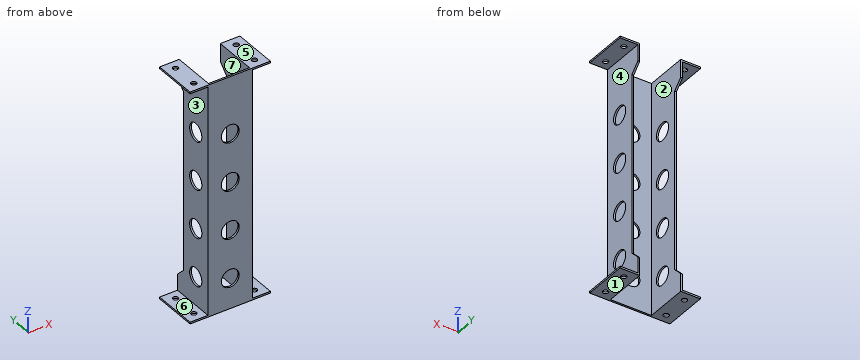
```python
from build123d import *

# Parameters (mm, degrees)
SKETCH1_W               = 25
SKETCH1_H               = 130
BOSS_EXTRUDE1_DEPTH     = 1
SKETCH2_W               = 1
SKETCH2_H               = 130
BOSS_EXTRUDE2_DEPTH     = 24
SKETCH3_W               = 1
SKETCH3_H               = 25
BOSS_EXTRUDE3_DEPTH     = 10
SKETCH4_W               = 1
SKETCH4_H               = 25
BOSS_EXTRUDE4_DEPTH     = 10
SKETCH5_R               = 5
CUT_EXTRUDE1_DEPTH      = 2
SKETCH10_R              = 1.5
CUT_EXTRUDE3_DEPTH      = 131
CUT_EXTRUDE4_DEPTH      = 11
CUT_EXTRUDE4_DEPTH_BACK = 36
SKETCH9_R               = 5
CUT_EXTRUDE2_DEPTH      = 36


with BuildPart() as part:
    # Sketch1 → Boss-Extrude1 (new body)
    with BuildSketch(Plane(origin=(0, 0, 0), x_dir=(1, 0, 0), z_dir=(0, 1, 0))):
        Rectangle(SKETCH1_W, SKETCH1_H)
    extrude(amount=BOSS_EXTRUDE1_DEPTH)

    # Sketch2 → Boss-Extrude2 (add)
    with BuildSketch(Plane(origin=(0, 1, 0), x_dir=(1, 0, 0), z_dir=(0, 1, 0))):
        with Locations((12, 0)):
            Rectangle(SKETCH2_W, SKETCH2_H)
        with Locations((-12, 0)):
            Rectangle(SKETCH2_W, SKETCH2_H)
    extrude(amount=BOSS_EXTRUDE2_DEPTH)

    # Sketch3 → Boss-Extrude3 (add)
    with BuildSketch(Plane(origin=(12.5, 0, 0), x_dir=(0, 0, -1), z_dir=(1, 0, 0))):
        with Locations((-64.5, 12.5)):
            Rectangle(SKETCH3_W, SKETCH3_H)
        with Locations((64.5, 12.5)):
            Rectangle(SKETCH3_W, SKETCH3_H)
    extrude(amount=BOSS_EXTRUDE3_DEPTH)

    # Sketch4 → Boss-Extrude4 (add)
    with BuildSketch(Plane.ZY.offset(12.5)):
        with Locations((-64.5, 12.5)):
            Rectangle(SKETCH4_W, SKETCH4_H)
        with Locations((64.5, 12.5)):
            Rectangle(SKETCH4_W, SKETCH4_H)
    extrude(amount=BOSS_EXTRUDE4_DEPTH)

    # Sketch5 → Cut-Extrude1 (cut, through all)
    with BuildSketch(Plane(origin=(0, 1, 0), x_dir=(1, 0, 0), z_dir=(0, 1, 0))):
        with Locations((0, -33)):
            Circle(SKETCH5_R)
        with Locations((0, -6)):
            Circle(SKETCH5_R)
        with Locations((0, 21)):
            Circle(SKETCH5_R)
        with Locations((0, 48)):
            Circle(SKETCH5_R)
    extrude(amount=-CUT_EXTRUDE1_DEPTH, mode=Mode.SUBTRACT)

    # Sketch10 → Cut-Extrude3 (cut, through all)
    with BuildSketch(Plane.XY.offset(65)):
        with Locations((17, 20)):
            Circle(SKETCH10_R)
        with Locations((17, 5)):
            Circle(SKETCH10_R)
        with Locations((-17, 20)):
            Circle(SKETCH10_R)
        with Locations((-17, 5)):
            Circle(SKETCH10_R)
    extrude(amount=-CUT_EXTRUDE3_DEPTH, mode=Mode.SUBTRACT)

    # Sketch11 → Cut-Extrude4 (cut, two sides)
    with BuildSketch(Plane(origin=(12.5, 0, 0), x_dir=(0, 0, -1), z_dir=(1, 0, 0))) as cut_extrude4_sk:
        Polygon((0, 25), (-55, 25), (-50, 20), (0, 20), align=None)
        Polygon((55, 25), (0, 25), (0, 20), (50, 20), align=None)
    extrude(amount=CUT_EXTRUDE4_DEPTH, mode=Mode.SUBTRACT)
    extrude(cut_extrude4_sk.sketch, amount=-CUT_EXTRUDE4_DEPTH_BACK, mode=Mode.SUBTRACT)

    # Sketch9 → Cut-Extrude2 (cut, through all)
    with BuildSketch(Plane(origin=(12.5, 0, 0), x_dir=(0, 0, -1), z_dir=(1, 0, 0))):
        with Locations((-33, 10)):
            Circle(SKETCH9_R)
        with Locations((-6, 10)):
            Circle(SKETCH9_R)
        with Locations((21, 10)):
            Circle(SKETCH9_R)
        with Locations((48, 10)):
            Circle(SKETCH9_R)
    extrude(amount=-CUT_EXTRUDE2_DEPTH, mode=Mode.SUBTRACT)


solid = part.part
```
Design review of the part built by this model. Coordinates are the model's own, in mm. Face numbers are marked on the shaded views. A direction names the side the tool comes from. Give positions to 0.01 mm unless a question says otherwise; leave off trailing zeros. Loops run counter-clockwise (first coordinate to the right, second up) from the corner with the lowest first, then second, coordinate; pieces in that order, holes last. Notation, with made-up numbers: M 69,32.25 L 126,32.25 A22 cw 126,54.25 Z; hole C 23,73.5 d1. An arc over 180 degrees is marked long. Return JSON: item names as keys, results as strings. Group by question number.
Item 1: Insertion check: pin 1 Ø0.5 at (x, z) = (-12, 3) entering from +Y; pin 2 Ø8 at (y, z) = (6, 10.5) entering from -X; pin 3 Ø8 at (y, z) = (6.5, -19) entering from +X; pin 4 Ø4 at (x, y) = (-17, 20) entering from +Z. Each pin has a flat end and moves straight along its axis. Give the tip position at first contact, or say it passes through.
Item 2: We need section C-C (z = -21). Give the boundary of the cut face in (x, y).
Item 3: Mouldability with a two-part tool opening along Z and no side actions: class the marked faces 1, 2 and 3 as released by +Z, released by -Z, zero draft, split by the parting line, or undercut.
Item 4: We need section A-A (y = 23.25). Give the boundary of the cut face in (x, z).
Item 5: For probe 1 along Y at (x, z) = (17, 64.3); probe 2 along Z at (x, y) = (0, 0.45); probe 3 along X at (y, z) = (21, 59.5), list the stretches that pass through material, from the lowest coordinate up.
Item 6: We need section B-B (x = 0). Give the boundary of the cut face in (y, z).
Item 7: We need section D-D (z = 44). Give the boundary of the cut face in (x, y), and give its area (3 significant figures).
Item 8: Tool access review of the marked faces 4, 5, 6 and 7: name each direction out of +Z, -Z, +X, -X, +Y, -Y from which nothing blocks a thin tool from reaching the whole face with its end or side.
Output:
{
 "1": {"pin 1": "stops at y = 20", "pin 2": "stops at x = -12.5", "pin 3": "stops at x = 12.5", "pin 4": "stops at z = 65"},
 "2": {"outline": "M -12.5,0 L -5,0 L -5,1 L -11.5,1 L -11.5,5 L -12.5,5 Z; M -12.5,15 L -11.5,15 L -11.5,20 L -12.5,20 Z; M 5,0 L 12.5,0 L 12.5,5 L 11.5,5 L 11.5,1 L 5,1 Z; M 11.5,15 L 12.5,15 L 12.5,20 L 11.5,20 Z"},
 "3": {"face 1": "released by -Z", "face 2": "zero draft", "face 3": "undercut"},
 "4": {"outline": "M -22.5,-65 L -11.5,-65 L -11.5,-53.25 L -12.5,-53.25 L -12.5,-64 L -22.5,-64 Z; M -22.5,64 L -12.5,64 L -12.5,53.25 L -11.5,53.25 L -11.5,65 L -22.5,65 Z; M 11.5,-65 L 22.5,-65 L 22.5,-64 L 12.5,-64 L 12.5,-53.25 L 11.5,-53.25 Z; M 11.5,53.25 L 12.5,53.25 L 12.5,64 L 22.5,64 L 22.5,65 L 11.5,65 Z"},
 "5": {"probe 1": "y = 0 to 3.5, 6.5 to 18.5, 21.5 to 25", "probe 2": "z = -65 to -53, -43 to -26, -16 to 1, 11 to 28, 38 to 65", "probe 3": "x = -12.5 to -11.5, 11.5 to 12.5"},
 "6": {"outline": "M 0,-65 L 1,-65 L 1,-53 L 0,-53 Z; M 0,-43 L 1,-43 L 1,-26 L 0,-26 Z; M 0,-16 L 1,-16 L 1,1 L 0,1 Z; M 0,11 L 1,11 L 1,28 L 0,28 Z; M 0,38 L 1,38 L 1,65 L 0,65 Z"},
 "7": {"outline": "M -12.5,0 L 12.5,0 L 12.5,20 L 11.5,20 L 11.5,1 L -11.5,1 L -11.5,20 L -12.5,20 Z", "area": "63.0 mm^2"},
 "8": {"face 4": "+X, +Y, -Y", "face 5": "+Z, +X, -X, +Y, -Y", "face 6": "-X, +Y, -Y", "face 7": "+Z, -Z, +Y"}
}
